For this review, take the finished solid that the model builds, in its own axes (mm). Face numbers are marked on the shaded views. A direction names the side the tool comes from. Round coordinates to 2 decimals unless told otherwise and drop trailing zeros. Order: outer loops, then holes, each group sorted by start corner. A loop starts at its lowest first (then second) coordinate and runs counter-clockwise, first axis right, second up. Notation, with made-up numbers: M 15.5,36.5 L 22.5,36.5 A35 cw 22.5,69.5 Z; hole C 3.5,44 d2. An arc over 180 degrees is marked long. Use a Markdown table: item, result.
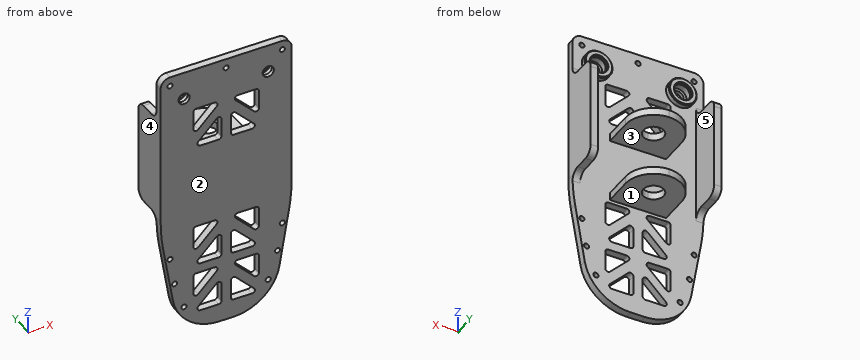
from build123d import *

# Parameters (mm, degrees)
EXTRUDE_1_DEPTH            = 8
EXTRUDE_START              = -100
EXTRUDE_3_DEPTH            = 80
SKETCH_5_W                 = 80
SKETCH_5_H                 = 60
CUT_EXTRUDE_2_DEPTH        = 110
FILLET_1_R                 = 50
FILLET_2_R                 = 200
SKETCH_7_R                 = 9
CUT_EXTRUDE_6_DEPTH        = 4
SKETCH_10_R                = 6
CUT_EXTRUDE_7_DEPTH        = 28
SKETCH_12_R                = 15
EXTRUDE_5_DEPTH            = 6
SKETCH_13_R                = 9
CUT_EXTRUDE_9_DEPTH        = 6
CUT_EXTRUDE_START          = -2.15
SKETCH_14_R                = 9.5
CUT_EXTRUDE_4235_DEPTH     = 1.1
CHAMFER_1_SIZE             = 1
CHAMFER_1_OF_MIRROR_1_SIZE = 1
SKETCH_23_W                = 8
SKETCH_23_H                = 110
EXTRUDE_7_DEPTH            = 35
FILLET_5_R                 = 10
MOVE_FACE_1_BY             = 2
MOVE_FACE_1_2_BY           = 2
SKETCH_24_R                = 2.75
CUT_EXTRUDE_13_DEPTH       = 40
FILLET_6_R                 = 3


with BuildPart() as part:
    # 草图1 → 凸台-拉伸1 (new body)
    with BuildSketch(Plane(origin=(0, 0, 0), x_dir=(1, 0, 0), z_dir=(0, 1, 0))):
        Polygon((-70, 0), (70, 0), (70, 180), (50, 300), (-50, 300), (-70, 180), align=None)
    extrude(amount=EXTRUDE_1_DEPTH)

    # 草图4 → 凸台-拉伸3 (add)
    with BuildSketch(Plane.XY.offset(EXTRUDE_START)):
        with BuildLine():
            Line((0, 27), (0, 8))
            Line((0, 8), (30, 8))
            Line((30, 8), (30, 38))
            ThreePointArc((30, 38), (21.213203436, 59.213203436), (0, 68))
            Line((0, 68), (0, 49))
            ThreePointArc((0, 49), (7.778174593, 45.778174593), (11, 38))
            ThreePointArc((11, 38), (7.778174593, 30.221825407), (0, 27))
        make_face()
        with BuildLine():
            Line((-30, 8), (0, 8))
            Line((0, 8), (0, 27))
            ThreePointArc((0, 27), (-11, 38), (0, 49))
            Line((0, 49), (0, 68))
            ThreePointArc((0, 68), (-21.213203436, 59.213203436), (-30, 38))
            Line((-30, 38), (-30, 8))
        make_face()
    extrude(amount=-EXTRUDE_3_DEPTH)

    # 草图5 → 切除-拉伸2 (cut)
    with BuildSketch(Plane(origin=(0, 8, 0), x_dir=(1, 0, 0), z_dir=(0, 1, 0))):
        with Locations((0, 140)):
            Rectangle(SKETCH_5_W, SKETCH_5_H)
    extrude(amount=CUT_EXTRUDE_2_DEPTH, mode=Mode.SUBTRACT)

    # 圆角1
    fillet_1_edges = [part.edges().sort_by_distance(p)[0] for p in [
        (-50, 4, -300),
        (50, 4, -300),
    ]]
    fillet(fillet_1_edges, radius=FILLET_1_R)

    # 圆角2
    fillet_2_edges = [part.edges().sort_by_distance(p)[0] for p in [
        (-70, 4, -180),
        (70, 4, -180),
    ]]
    fillet(fillet_2_edges, radius=FILLET_2_R)

    # 草图7 → 切除-拉伸6 (cut)
    with BuildSketch(Plane(origin=(0, 8, 0), x_dir=(1, 0, 0), z_dir=(0, 1, 0))):
        with Locations(Location((45, 30, 0), (0, 0, 270))):
            Circle(SKETCH_7_R)
    cut_extrude_6 = extrude(amount=-CUT_EXTRUDE_6_DEPTH, mode=Mode.SUBTRACT)

    # 草图10 → 切除-拉伸7 (cut)
    with BuildSketch(Plane(origin=(0, 4, 0), x_dir=(1, 0, 0), z_dir=(0, 1, 0))):
        with Locations(Location((45, 30, 0), (0, 0, 270))):
            Circle(SKETCH_10_R)
    cut_extrude_7 = extrude(amount=-CUT_EXTRUDE_7_DEPTH, mode=Mode.SUBTRACT)

    # 草图12 → 凸台-拉伸5 (add)
    with BuildSketch(Plane(origin=(0, 8, 0), x_dir=(1, 0, 0), z_dir=(0, 1, 0))):
        with Locations(Location((45, 30, 0), (0, 0, 270))):
            Circle(SKETCH_12_R)
    extrude_5 = extrude(amount=EXTRUDE_5_DEPTH)

    # 草图13 → 切除-拉伸9 (cut)
    with BuildSketch(Plane(origin=(0, 14, 0), x_dir=(1, 0, 0), z_dir=(0, 1, 0))):
        with Locations(Location((45, 30, 0), (0, 0, 270))):
            Circle(SKETCH_13_R)
    cut_extrude_9 = extrude(amount=-CUT_EXTRUDE_9_DEPTH, mode=Mode.SUBTRACT)

    # 草图14 → Cut-Extrude 4235 (cut)
    with BuildSketch(Plane(origin=(0, 14, 0), x_dir=(1, 0, 0), z_dir=(0, 1, 0)).offset(CUT_EXTRUDE_START)):
        with Locations(Location((45, 30, 0), (0, 0, 270))):
            Circle(SKETCH_14_R)
    cut_extrude_4235 = extrude(amount=-CUT_EXTRUDE_4235_DEPTH, mode=Mode.SUBTRACT)

    # 倒角1
    chamfer_1_edges = [part.edges().sort_by_distance(p)[0] for p in [
        (45, 14, -45),
        (45, 14, -39),
    ]]
    chamfer(chamfer_1_edges, length=CHAMFER_1_SIZE)

    # 镜向1: 切除-拉伸6, 切除-拉伸7, 凸台-拉伸5, 切除-拉伸9, Cut-Extrude 4235 across plane
    add(cut_extrude_6.mirror(Plane.ZY), mode=Mode.SUBTRACT)
    add(cut_extrude_7.mirror(Plane.ZY), mode=Mode.SUBTRACT)
    add(extrude_5.mirror(Plane.ZY))
    add(cut_extrude_9.mirror(Plane.ZY), mode=Mode.SUBTRACT)
    add(cut_extrude_4235.mirror(Plane.ZY), mode=Mode.SUBTRACT)

    # 倒角1 of 镜向1
    chamfer_1_of_mirror_1_edges = [part.edges().sort_by_distance(p)[0] for p in [
        (-45, 14, -45),
        (-45, 14, -39),
    ]]
    chamfer(chamfer_1_of_mirror_1_edges, length=CHAMFER_1_OF_MIRROR_1_SIZE)

    # 草图23 → 凸台-拉伸7 (add)
    with BuildSketch(Plane(origin=(0, 8, 0), x_dir=(1, 0, 0), z_dir=(0, 1, 0))):
        with Locations((66, 105)):
            Rectangle(SKETCH_23_W, SKETCH_23_H)
        with Locations((-66, 105)):
            Rectangle(SKETCH_23_W, SKETCH_23_H)
    extrude(amount=EXTRUDE_7_DEPTH)

    # 圆角5
    fillet_5_edges = [part.edges().sort_by_distance(p)[0] for p in [
        (70, 4, 0),
        (-70, 4, 0),
        (66, 8, -50),
        (66, 8, -160),
        (66, 43, -50),
        (66, 43, -160),
        (-66, 8, -160),
        (-66, 8, -50),
        (-66, 43, -160),
        (-66, 43, -50),
    ]]
    fillet(fillet_5_edges, radius=FILLET_5_R)

    # Move Face 1: a face moved inward by 2.0
    extrude(part.faces().sort_by_distance((0, 23, -180))[0], amount=MOVE_FACE_1_BY, dir=(0, 0, 1), mode=Mode.SUBTRACT)

    # Move Face 1 2: a face moved inward by 2.0
    extrude(part.faces().sort_by_distance((0, 23, -100))[0], amount=MOVE_FACE_1_2_BY, dir=(0, 0, -1), mode=Mode.SUBTRACT)

    # 草图24 → 切除-拉伸13 (cut)
    with BuildSketch(Plane(origin=(0, 8, 0), x_dir=(1, 0, 0), z_dir=(0, 1, 0))):
        with Locations(Location((45, 270, 0), (0, 0, 270))):
            Circle(SKETCH_24_R)
        with Locations(Location((55, 240, 0), (0, 0, 270))):
            Circle(SKETCH_24_R)
        with Locations(Location((60, 210, 0), (0, 0, 270))):
            Circle(SKETCH_24_R)
        with Locations(Location((60, 10, 0), (0, 0, 270))):
            Circle(SKETCH_24_R)
        with Locations(Location((0, 10, 0), (0, 0, 270))):
            Circle(SKETCH_24_R)
        with Locations(Location((-60, 10, 0), (0, 0, 270))):
            Circle(SKETCH_24_R)
        with Locations(Location((-60, 210, 0), (0, 0, 270))):
            Circle(SKETCH_24_R)
        with Locations(Location((-55, 240, 0), (0, 0, 270))):
            Circle(SKETCH_24_R)
        with Locations(Location((-45, 270, 0), (0, 0, 270))):
            Circle(SKETCH_24_R)
        Polygon((5, 90), (35, 90), (5, 60), align=None)
        Polygon((35, 75.857864376), (5, 45.857864376), (35, 45.857864376), align=None)
        Polygon((-5, 45.857864376), (-35, 45.857864376), (-35, 75.857864376), align=None)
        Polygon((-35, 90), (-5, 60), (-5, 90), align=None)
        Polygon((5, 280), (35, 280), (5, 250), align=None)
        Polygon((35, 265.857864376), (5, 235.857864376), (35, 235.857864376), align=None)
        Polygon((5, 225.857864376), (35, 225.857864376), (5, 195.857864376), align=None)
        Polygon((35, 211.715728753), (5, 181.715728753), (35, 181.715728753), align=None)
        Polygon((-35, 181.715728753), (-35, 211.715728753), (-5, 181.715728753), align=None)
        Polygon((-5, 195.857864376), (-5, 225.857864376), (-35, 225.857864376), align=None)
        Polygon((-35, 235.857864376), (-35, 265.857864376), (-5, 235.857864376), align=None)
        Polygon((-5, 250), (-5, 280), (-35, 280), align=None)
    extrude(amount=-CUT_EXTRUDE_13_DEPTH, mode=Mode.SUBTRACT)

    # 圆角6
    fillet_6_edges = [part.edges().sort_by_distance(p)[0] for p in [
        (-35, 4, -90),
        (-5, 4, -90),
        (-5, 4, -60),
        (5, 4, -250),
        (5, 4, -280),
        (35, 4, -280),
        (35, 4, -265.857864376),
        (35, 4, -235.857864376),
        (5, 4, -235.857864376),
        (35, 4, -75.857864376),
        (35, 4, -45.857864376),
        (5, 4, -45.857864376),
        (-35, 4, -75.857864376),
        (-5, 4, -45.857864376),
        (-35, 4, -45.857864376),
        (-5, 4, -235.857864376),
        (-35, 4, -235.857864376),
        (-35, 4, -265.857864376),
        (-5, 4, -250),
        (-35, 4, -280),
        (-5, 4, -280),
        (-5, 4, -181.715728753),
        (-35, 4, -181.715728753),
        (-35, 4, -211.715728753),
        (5, 4, -195.857864376),
        (5, 4, -225.857864376),
        (35, 4, -225.857864376),
        (35, 4, -211.715728753),
        (35, 4, -181.715728753),
        (5, 4, -181.715728753),
        (-5, 4, -195.857864376),
        (-35, 4, -225.857864376),
        (-5, 4, -225.857864376),
        (5, 4, -60),
        (5, 4, -90),
        (35, 4, -90),
    ]]
    fillet(fillet_6_edges, radius=FILLET_6_R)


solid = part.part
Q1. Draft analysis for pull direction Z (two halves, no side actions). For the marked faces 1, 2 and 3, state which applies: pulls with the +Z half, pulls with the -Z half, needs draft (parallel to the pull), parting line crosses it, or undercut.
Determined:
| item | result |
|---|---|
| face 1 | pulls with the -Z half |
| face 2 | needs draft |
| face 3 | undercut |
Q2. Clearance check with flat-ended pins moving along their axes: pin 1 (4 mm diameter, centred on x = 65, z = -95, fed in from +Y); pin 2 (9.5 mm diameter, centred on x = 41, z = -29.5, fed in from +Y); pin 3 (2.5 mm diameter, centred on y = 16, z = -175.5, fed in from +X). State where each tip first meets the part, or that it passes through.
Determined:
| item | result |
|---|---|
| pin 1 | stops at y = 43 |
| pin 2 | stops at y = 4 |
| pin 3 | stops at x = 30 |
Q3. Add section A-A (y = 21). Write out the cut boundary in (x, z), then the cut area to 3 significant figures.
Determined:
| item | result |
|---|---|
| outline | M -70,-160 L -62,-160 L -62,-50 L -70,-50 Z; M -30,-178 L 30,-178 L 30,-170 L -30,-170 Z; M -30,-110 L 30,-110 L 30,-102 L -30,-102 Z; M 62,-160 L 70,-160 L 70,-50 L 62,-50 Z |
| area | 2,720 mm^2 |
Q4. Add section C-C (x = 45). Give the number of separate pieces and of enclosed holes in the cut face, then the cut area to 3 significant figures.
Determined:
| item | result |
|---|---|
| separate pieces | 3 |
| enclosed holes | 0 |
| area | 2,170 mm^2 |
Q5. Add section D-D (y = 57). Write out the cut boundary in (x, z).
Determined:
| item | result |
|---|---|
| outline | M -23.22,-178 L 23.22,-178 L 23.22,-170 L -23.22,-170 Z; M -23.22,-110 L 23.22,-110 L 23.22,-102 L -23.22,-102 Z |
Q6. Wall thickness on line 1 along X through (y, z) = (11.25, -30); line 2 along X through (y, z) = (12.2, -30); line 3 along Z through (x, y) = (20.5, 13): over which ranges is each line inside the solid? List them lowest first. Write a range as [from, to].
Determined:
| item | result |
|---|---|
| line 1 | x = [-60, -54.5], [-35.5, -30], [30, 35.5], [54.5, 60] |
| line 2 | x = [-60, -54], [-36, -30], [30, 36], [54, 60] |
| line 3 | z = [-178, -170], [-110, -102] |
Q7. Machinability: for the marked faces 4 and 5, which of the approach directions +Z, -Z, +X, -X, +Y, -Y give a long, thin tool a straight path to every point of the face, cutting with its end or side? Answer none if there is none.
Determined:
| item | result |
|---|---|
| face 4 | +Z, -Z, -X, +Y, -Y |
| face 5 | +Z, -Z, +Y |
Q8. Add section B-B (z = -246). Write out the cut boundary in (x, y), then the cut area to 3 significant figures.
Determined:
| item | result |
|---|---|
| outline | M -59,0 L -35,0 L -35,8 L -59,8 Z; M -15.14,0 L 15.14,0 L 15.14,8 L -15.14,8 Z; M 35,0 L 59,0 L 59,8 L 35,8 Z |
| area | 626 mm^2 |
